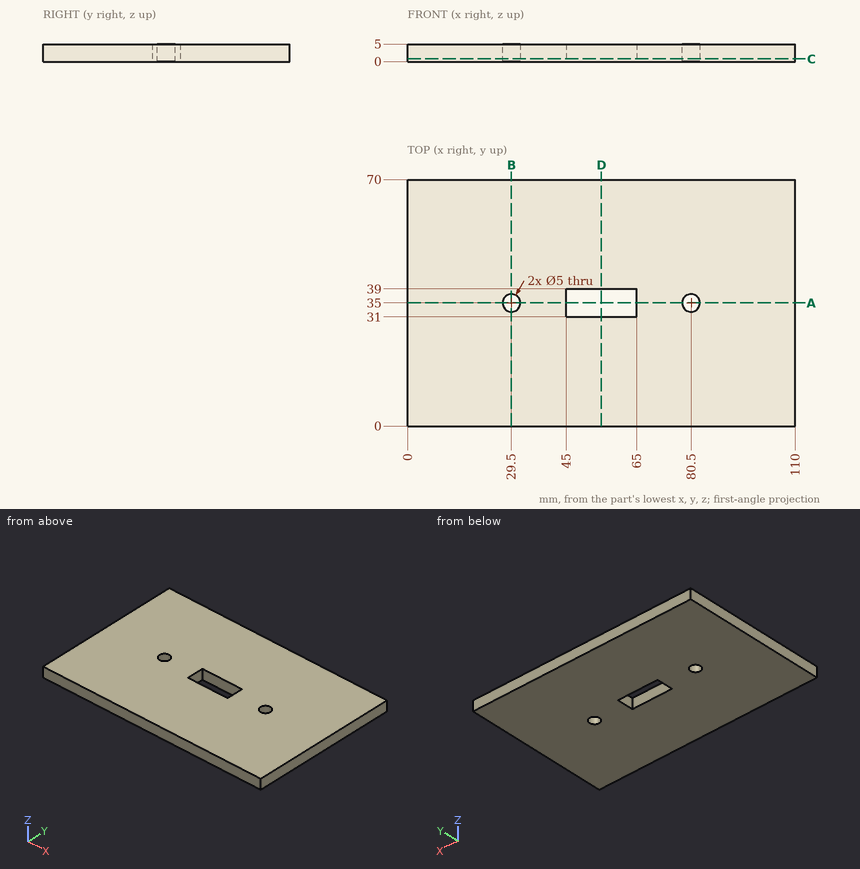
Check sheet for the drawn part. Datum: minimum x, y, z corner. Units: mm. Round coordinates to 2 decimals unless told otherwise and drop trailing zeros. Write each loop counter-clockwise with the first axis right and the second up, starting at its lowest first coordinate (ties: lowest second). Pieces come first, ordered by that corner, then holes. Notation, with made-up numbers: (-8, 14) -> (40, 14) arc R20 ccw to (40, 51) -> close; hole circle Ø8 at (67, 1.25). An arc over 180 degrees is marked (long way). One line per item, written item: value. Start each with the question number.
(1) Scan lines: line 1 (Y direction, x = 29.5, z = 2.35); line 2 (X direction, y = 34, z = 2.2); line 3 (X direction, y = 31.5, z = 0.7). Record each from-to range of solid material in increasing order. Write a range as [from, to].
(2) Cross-section at A-A, the plane y = 35. Record the cut outline in (x, z).
(3) Cross-section at C-C, the plane z = 0.8. Record the cut outline in (x, y), and give its area (3 significant figures).
(4) Cross-section at D-D, the plane x = 55. Record the cut outline in (y, z).
(5) Cross-section at B-B, the plane x = 29.5. Record the cut outline in (y, z).
(6) Go/stop test with flat-tipped pins: pin 1 Ø4.5 at (x, y) = (29.5, 35) entering from -Z; pin 2 Ø10 at (x, y) = (18, 41) entering from -Z. Record where each tip stops, or that it passes through.
Answer:
1. line 1: [0, 32.5], [37.5, 70]
1. line 2: [0, 27.21], [31.79, 45], [65, 78.21], [82.79, 110]
1. line 3: [0, 45], [65, 110]
2. outline: (0, 0) -> (27, 0) -> (27, 5) -> (0, 5) -> close; (32, 0) -> (45, 0) -> (45, 5) -> (32, 5) -> close; (65, 0) -> (78, 0) -> (78, 5) -> (65, 5) -> close; (83, 0) -> (110, 0) -> (110, 5) -> (83, 5) -> close
3. outline: (0, 0) -> (110, 0) -> (110, 70) -> (0, 70) -> close; hole circle Ø5 at (29.5, 35); hole (45, 31) -> (65, 31) -> (65, 39) -> (45, 39) -> close; hole circle Ø5 at (80.5, 35)
3. area: 7,500 mm²
4. outline: (0, 0) -> (31, 0) -> (31, 5) -> (0, 5) -> close; (39, 0) -> (70, 0) -> (70, 5) -> (39, 5) -> close
5. outline: (0, 0) -> (32.5, 0) -> (32.5, 5) -> (0, 5) -> close; (37.5, 0) -> (70, 0) -> (70, 5) -> (37.5, 5) -> close
6. pin 1: through
6. pin 2: z = 0
